Build history of the part. All positions in model axes, mm. A direction names the side the tool comes from. Round coordinates to 2 decimals unless told otherwise and drop trailing zeros. Write each loop counter-clockwise with the first axis right and the second up, starting at its lowest first coordinate (ties: lowest second). Pieces come first, ordered by that corner, then holes. Notation, with made-up numbers: M -14.75,2 L 31.25,2 A32 ccw 31.25,33 Z; hole C -34.75,68 d5. An arc over 180 degrees is marked long. Use a Markdown table: item, result.
from build123d import *

# Parameters (mm, degrees)
F0_W     = 250
F0_H     = 200
F1_DEPTH = 150
F2_T     = -2.5
F3_R     = 1.29


with BuildPart() as f1:
    # F0 (on Top) → F1 (new body)
    with BuildSketch(Plane.XY):
        with Locations((125, 100)):
            Rectangle(F0_W, F0_H)
    extrude(amount=F1_DEPTH)

    # F2
    f2_openings = [f1.faces().sort_by_distance(p)[0] for p in [
        (125, 100, 150),
    ]]
    offset(amount=F2_T, openings=f2_openings)

    # F3
    f3_edges = [f1.edges().sort_by_distance(p)[0] for p in [
        (2.5, 100, 2.5),
        (125, 197.5, 2.5),
        (247.5, 100, 2.5),
        (125, 2.5, 2.5),
    ]]
    fillet(f3_edges, radius=F3_R)


solid = f1.part
Q1. Which spindle directions (+Z, -Z, +X, -X, +Y, -Y) get a long thin tool onto all of the face, cutting with end or side? Do faces 5 (the flat face through (123, 101, 2.5)), 6 (the flat face through (123, 0, 74)). Say none if no direction does.
Response values:
| item | result |
|---|---|
| face 5 | +Z |
| face 6 | +Z, -Z, +X, -X, -Y |
Q2. Cut at A-A on z = 104. Give the cut face in (x, y).
Response values:
| item | result |
|---|---|
| outline | M 0,0 L 250,0 L 250,200 L 0,200 Z; hole M 2.5,2.5 L 247.5,2.5 L 247.5,197.5 L 2.5,197.5 Z |
Q3. Drill centre lines: L1, parallel to Y at x = 125.5, z = 125.5; L2, parallel to X at y = 140, z = 61.5; L3, parallel to Z at x = 219.5, y = 10. Where is each one in solid material? Low to high.
Response values:
| item | result |
|---|---|
| L1 | y = 0 to 2.5, 197.5 to 200 |
| L2 | x = 0 to 2.5, 247.5 to 250 |
| L3 | z = 0 to 2.5 |
Q4. Cut at C-C on x = 67. Give the cut face in (y, z).
Response values:
| item | result |
|---|---|
| outline | M 0,0 L 200,0 L 200,150 L 197.5,150 L 197.5,3.79 A1.29 cw 196.21,2.5 L 3.79,2.5 A1.29 cw 2.5,3.79 L 2.5,150 L 0,150 Z |
Q5. Cut at B-B on y = 22. Give the cut face in (x, z).
Response values:
| item | result |
|---|---|
| outline | M 0,0 L 250,0 L 250,150 L 247.5,150 L 247.5,3.79 A1.29 cw 246.21,2.5 L 3.79,2.5 A1.29 cw 2.5,3.79 L 2.5,150 L 0,150 Z |
Q6. Two-plate mould, pull along Y, no slides. Class faces 1 (the flat face through (123, 197.5, 76)), 2 (the flat face through (123, 200, 74)), 3 (the flat face through (0, 99, 74)), 4 (the flat face through (123, 2.5, 76)): +Y half, -Y half, draft (parallel to the pull), parting line (faces both ways), or undercut.
Response values:
| item | result |
|---|---|
| face 1 | undercut |
| face 2 | +Y half |
| face 3 | draft |
| face 4 | undercut |
